Model file for the job. Use its own axes, mm. Face numbers are marked on the shaded views. A direction names the side the tool comes from. Give positions to 0.01 mm unless a question says otherwise; leave off trailing zeros. Order: outer loops, then holes, each group sorted by start corner. A loop starts at its lowest first (then second) coordinate and runs counter-clockwise, first axis right, second up. Notation, with made-up numbers: M -8,-4.75 L 49,-4.75 A24 ccw 49,9.25 Z; hole C 62,38 d3. An arc over 180 degrees is marked long. Return JSON: item names as keys, results as strings. Group by question number.
1. 3-axis set-ups, long thin cutter, end or side, ignore diameter. For the marked faces 4 and 5: which of +Z, -Z, +X, -X, +Y, -Y reach the whole face in a straight line?
2. Slice it at A-A on z = 6.35. List the corners of the cut face in (x, y) (3 decimals), then the cut area to 3 significant figures.
3. Slice it at D-D on y = 11. List the corners of the cut face in (x, z) (1 decimal), then the cut area to 3 significant figures.
4. Slice it at B-B on x = -0.5. List the corners of the cut face in (y, z).
5. Slice it at C-C on x = 2.25. List the corners of the cut face in (y, z), then the cut area to 3 significant figures.
6. Wall check: probe 1 along X at (y, z) = (24.5, 10.5) (3 decimals); probe 2 along Y at (x, z) = (-1.7, 6.35); probe 3 along Y at (x, z) = (-0.85, 6.35). Give the ranges that are in metal, low to high. Write a range as [from, to].
7. Two-plate mould, pull along Z, no slides. Class the marked faces 1, 2 and 3: released by +Z, released by -Z, zero draft, split by the parting line, or undercut.
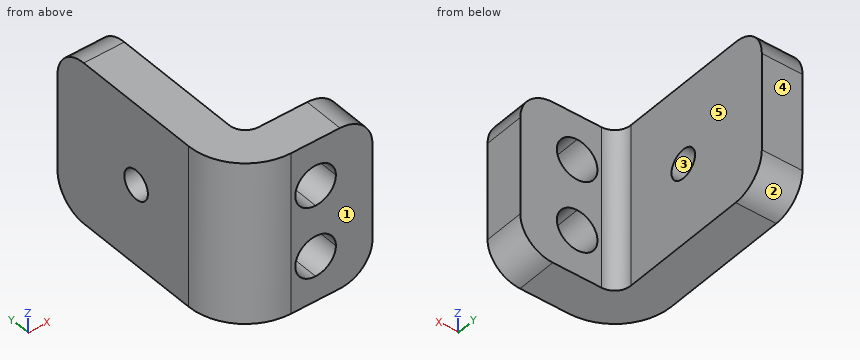
from build123d import *

# Parameters (mm, degrees)
BOSS_EXTRUDE1_DEPTH = 12.7
FILLET1_R           = 2.54
SKETCH2_R           = 1.143
CUT_EXTRUDE1_DEPTH  = 3.175
CUT_EXTRUDE2_REACH  = 22.36


with BuildPart() as part:
    # Sketch1 → Boss-Extrude1 (new body)
    with BuildSketch(Plane.XY):
        with BuildLine():
            Line((0, 25.690786623), (0, 12.990786623))
            ThreePointArc((0, 12.990786623), (0.371974388, 12.092761011), (1.27, 11.720786623))
            Line((1.27, 11.720786623), (7.62, 11.720786623))
            Line((7.62, 11.720786623), (7.62, 8.545786623))
            Line((7.62, 8.545786623), (1.27, 8.545786623))
            ThreePointArc((1.27, 8.545786623), (-1.873089642, 9.847696981), (-3.175, 12.990786623))
            Line((-3.175, 12.990786623), (-3.175, 25.690786623))
            Line((-3.175, 25.690786623), (0, 25.690786623))
        make_face()
    extrude(amount=BOSS_EXTRUDE1_DEPTH)

    # Fillet1
    fillet1_edges = [part.edges().sort_by_distance(p)[0] for p in [
        (-1.5875, 25.690786623, 0),
        (7.62, 10.133286623, 12.7),
        (-1.5875, 25.690786623, 12.7),
        (7.62, 10.133286623, 0),
    ]]
    fillet(fillet1_edges, radius=FILLET1_R)

    # Sketch2 → Cut-Extrude1 (cut)
    with BuildSketch(Plane(origin=(0, 0, 0), x_dir=(0, 0, -1), z_dir=(1, 0, 0))):
        with Locations((-6.35, 18.070786623)):
            Circle(SKETCH2_R)
    extrude(amount=-CUT_EXTRUDE1_DEPTH, mode=Mode.SUBTRACT)

    # Sketch3 → Cut-Extrude2 (cut, up to next)
    with BuildSketch(Plane(origin=(0, 11.720786623, 0), x_dir=(1, 0, 0), z_dir=(0, 1, 0)), mode=Mode.PRIVATE) as cut_extrude2_sk1:
        with BuildLine():
            ThreePointArc((3.175, -7.5565), (1.5875, -9.144), (3.175, -10.7315))
            Line((3.175, -10.7315), (3.175, -7.5565))
        make_face()
    cut_extrude2_tool1 = extrude(cut_extrude2_sk1.sketch, amount=-CUT_EXTRUDE2_REACH, mode=Mode.PRIVATE) & part.part
    # Sketch3 → Cut-Extrude2 (cut, up to next)
    with BuildSketch(Plane(origin=(0, 11.720786623, 0), x_dir=(1, 0, 0), z_dir=(0, 1, 0)), mode=Mode.PRIVATE) as cut_extrude2_sk2:
        with BuildLine():
            Line((3.175, -7.5565), (3.175, -10.7315))
            ThreePointArc((3.175, -10.7315), (4.297532015, -10.266532015), (4.7625, -9.144))
            ThreePointArc((4.7625, -9.144), (4.297532015, -8.021467985), (3.175, -7.5565))
        make_face()
    cut_extrude2_tool2 = extrude(cut_extrude2_sk2.sketch, amount=-CUT_EXTRUDE2_REACH, mode=Mode.PRIVATE) & part.part
    # Sketch3 → Cut-Extrude2 (cut, up to next)
    with BuildSketch(Plane(origin=(0, 11.720786623, 0), x_dir=(1, 0, 0), z_dir=(0, 1, 0)), mode=Mode.PRIVATE) as cut_extrude2_sk3:
        with BuildLine():
            ThreePointArc((3.175, -7.5565), (1.5875, -9.144), (3.175, -10.7315))
            Line((3.175, -10.7315), (3.175, -7.5565))
        make_face()
    cut_extrude2_tool3 = extrude(cut_extrude2_sk3.sketch, amount=-CUT_EXTRUDE2_REACH, mode=Mode.PRIVATE) & part.part
    # Sketch3 → Cut-Extrude2 (cut, up to next)
    with BuildSketch(Plane(origin=(0, 11.720786623, 0), x_dir=(1, 0, 0), z_dir=(0, 1, 0)), mode=Mode.PRIVATE) as cut_extrude2_sk4:
        with BuildLine():
            Line((3.175, -7.5565), (3.175, -10.7315))
            ThreePointArc((3.175, -10.7315), (4.297532015, -10.266532015), (4.7625, -9.144))
            ThreePointArc((4.7625, -9.144), (4.297532015, -8.021467985), (3.175, -7.5565))
        make_face()
    cut_extrude2_tool4 = extrude(cut_extrude2_sk4.sketch, amount=-CUT_EXTRUDE2_REACH, mode=Mode.PRIVATE) & part.part
    # Sketch3 → Cut-Extrude2 (cut, up to next)
    with BuildSketch(Plane(origin=(0, 11.720786623, 0), x_dir=(1, 0, 0), z_dir=(0, 1, 0)), mode=Mode.PRIVATE) as cut_extrude2_sk5:
        with BuildLine():
            ThreePointArc((3.175, -1.9685), (1.5875, -3.556), (3.175, -5.1435))
            Line((3.175, -5.1435), (3.175, -1.9685))
        make_face()
    cut_extrude2_tool5 = extrude(cut_extrude2_sk5.sketch, amount=-CUT_EXTRUDE2_REACH, mode=Mode.PRIVATE) & part.part
    # Sketch3 → Cut-Extrude2 (cut, up to next)
    with BuildSketch(Plane(origin=(0, 11.720786623, 0), x_dir=(1, 0, 0), z_dir=(0, 1, 0)), mode=Mode.PRIVATE) as cut_extrude2_sk6:
        with BuildLine():
            Line((3.175, -1.9685), (3.175, -5.1435))
            ThreePointArc((3.175, -5.1435), (4.297532015, -4.678532015), (4.7625, -3.556))
            ThreePointArc((4.7625, -3.556), (4.297532015, -2.433467985), (3.175, -1.9685))
        make_face()
    cut_extrude2_tool6 = extrude(cut_extrude2_sk6.sketch, amount=-CUT_EXTRUDE2_REACH, mode=Mode.PRIVATE) & part.part
    # Sketch3 → Cut-Extrude2 (cut, up to next)
    with BuildSketch(Plane(origin=(0, 11.720786623, 0), x_dir=(1, 0, 0), z_dir=(0, 1, 0)), mode=Mode.PRIVATE) as cut_extrude2_sk7:
        with BuildLine():
            ThreePointArc((3.175, -1.9685), (1.5875, -3.556), (3.175, -5.1435))
            Line((3.175, -5.1435), (3.175, -1.9685))
        make_face()
    cut_extrude2_tool7 = extrude(cut_extrude2_sk7.sketch, amount=-CUT_EXTRUDE2_REACH, mode=Mode.PRIVATE) & part.part
    # Sketch3 → Cut-Extrude2 (cut, up to next)
    with BuildSketch(Plane(origin=(0, 11.720786623, 0), x_dir=(1, 0, 0), z_dir=(0, 1, 0)), mode=Mode.PRIVATE) as cut_extrude2_sk8:
        with BuildLine():
            Line((3.175, -1.9685), (3.175, -5.1435))
            ThreePointArc((3.175, -5.1435), (4.297532015, -4.678532015), (4.7625, -3.556))
            ThreePointArc((4.7625, -3.556), (4.297532015, -2.433467985), (3.175, -1.9685))
        make_face()
    cut_extrude2_tool8 = extrude(cut_extrude2_sk8.sketch, amount=-CUT_EXTRUDE2_REACH, mode=Mode.PRIVATE) & part.part
    add(cut_extrude2_tool1.solids().sort_by_distance((2.501244, 11.720787, 9.144))[0], mode=Mode.SUBTRACT)
    add(cut_extrude2_tool2.solids().sort_by_distance((3.848756, 11.720787, 9.144))[0], mode=Mode.SUBTRACT)
    add(cut_extrude2_tool3.solids().sort_by_distance((2.501244, 11.720787, 9.144))[0], mode=Mode.SUBTRACT)
    add(cut_extrude2_tool4.solids().sort_by_distance((3.848756, 11.720787, 9.144))[0], mode=Mode.SUBTRACT)
    add(cut_extrude2_tool5.solids().sort_by_distance((2.501244, 11.720787, 3.556))[0], mode=Mode.SUBTRACT)
    add(cut_extrude2_tool6.solids().sort_by_distance((3.848756, 11.720787, 3.556))[0], mode=Mode.SUBTRACT)
    add(cut_extrude2_tool7.solids().sort_by_distance((2.501244, 11.720787, 3.556))[0], mode=Mode.SUBTRACT)
    add(cut_extrude2_tool8.solids().sort_by_distance((3.848756, 11.720787, 3.556))[0], mode=Mode.SUBTRACT)


solid = part.part
Result:
{
 "1": {"face 4": "+Z, -Z, +X, -X, +Y", "face 5": "+Z, -Z, +X, +Y"},
 "2": {"outline": "M -3.175,12.991 A4.445 ccw 1.27,8.546 L 7.62,8.546 L 7.62,11.721 L 1.27,11.721 A1.27 cw 0,12.991 L 0,16.928 L -3.175,16.928 Z; M -3.175,19.214 L 0,19.214 L 0,25.691 L -3.175,25.691 Z", "area": "67.5 mm2"},
 "3": {"outline": "M -2.7,0 L 5.1,0 A2.5 ccw 7.6,2.5 L 7.6,10.2 A2.5 ccw 5.1,12.7 L -2.7,12.7 Z; hole C 3.2,3.6 d3.2; hole C 3.2,9.1 d3.2", "area": "113 mm2"},
 "4": {"outline": "M 8.91,0 L 23.15,0 A2.54 ccw 25.69,2.54 L 25.69,10.16 A2.54 ccw 23.15,12.7 L 8.91,12.7 Z; hole C 18.07,6.35 d2.29"},
 "5": {"outline": "M 8.55,0 L 11.72,0 L 11.72,2.27 L 8.55,2.27 Z; M 8.55,4.85 L 11.72,4.85 L 11.72,7.85 L 8.55,7.85 Z; M 8.55,10.43 L 11.72,10.43 L 11.72,12.7 L 8.55,12.7 Z", "area": "23.9 mm2"},
 "6": {"probe 1": "x = [-3.175, 0]", "probe 2": "y = [9.68, 16.93], [19.21, 25.69]", "probe 3": "y = [9.08, 16.93], [19.21, 25.69]"},
 "7": {"face 1": "zero draft", "face 2": "released by -Z", "face 3": "undercut"}
}
